```python
from build123d import *

# Parameters (mm, degrees)
SKETCH1_W                    = 443
SKETCH1_H                    = 300
BASE_FLANGE1_DEPTH           = 2
SKETCHED_START               = -221.5
SKETCHED_BEND1_DEPTH         = 443
SKETCHED_BEND1_2_DEPTH       = 443
SKETCHED_BEND2_DEPTH         = 443
SKETCHED_BEND2_2_DEPTH       = 443
EDGE_FLANGE1_STRIP_W         = 10
EDGE_FLANGE1_STRIP_H         = 2
EDGE_FLANGE1_STRIP_CUT_DEPTH = 238.429203673
EDGE_FLANGE1_DEPTH           = 238.429203673
EDGE_FLANGE2_STRIP_W         = 10
EDGE_FLANGE2_STRIP_H         = 2
EDGE_FLANGE2_STRIP_CUT_DEPTH = 238.429203673
EDGE_FLANGE2_DEPTH           = 238.429203673
SKETCH15_W                   = 420
SKETCH15_H                   = 165
CUT_EXTRUDE1_DEPTH           = 272.023210126


# Read off the part's stored shape, not the designer's step: Sketched Bend1, Sketched Bend2
# Sheet-metal steps are written as plain solids
with BuildPart() as part:
    # Sketch1 → Base-Flange1 (new body)
    with BuildSketch(Plane.XY):
        Rectangle(SKETCH1_W, SKETCH1_H)
    extrude(amount=-BASE_FLANGE1_DEPTH)

    # Sketched Bend1 outline → Sketched Bend1 (cut)
    with BuildSketch(Plane.YZ.offset(SKETCHED_START)):
        with BuildLine():
            Line((150, 0), (91.257630798, 0))
            ThreePointArc((91.257630798, 0), (90.161254481, -1.449489743), (88.429203673, -2))
            Line((88.429203673, -2), (150, -2))
            Line((150, -2), (150, 0))
        make_face()
    extrude(amount=SKETCHED_BEND1_DEPTH, mode=Mode.SUBTRACT)

    # Sketched Bend1 2 outline → Sketched Bend1 2 (add)
    with BuildSketch(Plane.YZ.offset(SKETCHED_START)):
        with BuildLine():
            Line((91.429203673, 1), (91.429203673, 59.429203673))
            Line((91.429203673, 59.429203673), (89.429203673, 59.429203673))
            Line((89.429203673, 59.429203673), (89.429203673, 1))
            ThreePointArc((89.429203673, 1), (89.136310454, 0.292893219), (88.429203673, 0))
            Line((88.429203673, 0), (91.257630798, 0))
            ThreePointArc((91.257630798, 0), (91.385999352, 0.492694064), (91.429203673, 1))
        make_face()
    extrude(amount=SKETCHED_BEND1_2_DEPTH)

    # Sketched Bend2 outline → Sketched Bend2 (cut)
    with BuildSketch(Plane.YZ.offset(SKETCHED_START)):
        with BuildLine():
            ThreePointArc((89.429203673, 31.472232635), (90.878693416, 30.375856318), (91.429203673, 28.64380551))
            Line((91.429203673, 28.64380551), (91.429203673, 59.429203673))
            Line((91.429203673, 59.429203673), (89.429203673, 59.429203673))
            Line((89.429203673, 59.429203673), (89.429203673, 31.472232635))
        make_face()
    extrude(amount=SKETCHED_BEND2_DEPTH, mode=Mode.SUBTRACT)

    # Sketched Bend2 2 outline → Sketched Bend2 2 (add)
    with BuildSketch(Plane.YZ.offset(SKETCHED_START)):
        with BuildLine():
            Line((89.429203673, 28.64380551), (89.429203673, 31.472232635))
            ThreePointArc((89.429203673, 31.472232635), (88.936509609, 31.600601189), (88.429203673, 31.64380551))
            Line((88.429203673, 31.64380551), (60.785398163, 31.64380551))
            Line((60.785398163, 31.64380551), (60.785398163, 29.64380551))
            Line((60.785398163, 29.64380551), (88.429203673, 29.64380551))
            ThreePointArc((88.429203673, 29.64380551), (89.136310454, 29.350912291), (89.429203673, 28.64380551))
        make_face()
    extrude(amount=SKETCHED_BEND2_2_DEPTH)

    # Edge-Flange1 strip (across the edge) → Edge-Flange1 strip cut (cut)
    with BuildSketch(Plane(origin=(-221.5, 88.429203673, 0), x_dir=(1, 0, 0), z_dir=(0, -1, 0))):
        with Locations((-4, -1)):
            Rectangle(EDGE_FLANGE1_STRIP_W, EDGE_FLANGE1_STRIP_H)
    extrude(amount=EDGE_FLANGE1_STRIP_CUT_DEPTH, mode=Mode.SUBTRACT)

    # Edge-Flange1 section (across the edge) → Edge-Flange1 (add)
    with BuildSketch(Plane(origin=(-221.5, 88.429203673, 0), x_dir=(1, 0, 0), z_dir=(0, -1, 0))):
        with BuildLine():
            Line((-2, 1), (-2, 10))
            Line((-2, 10), (0, 10))
            Line((0, 10), (0, 1))
            ThreePointArc((0, 1), (0.292893219, 0.292893219), (1, 0))
            Line((1, 0), (1, -2))
            ThreePointArc((1, -2), (-1.121320344, -1.121320344), (-2, 1))
        make_face()
    extrude(amount=EDGE_FLANGE1_DEPTH)

    # Edge-Flange2 strip (across the edge) → Edge-Flange2 strip cut (cut)
    with BuildSketch(Plane(origin=(221.5, -150, 0), x_dir=(-1, 0, 0), z_dir=(0, 1, 0))):
        with Locations((-4, -1)):
            Rectangle(EDGE_FLANGE2_STRIP_W, EDGE_FLANGE2_STRIP_H)
    extrude(amount=EDGE_FLANGE2_STRIP_CUT_DEPTH, mode=Mode.SUBTRACT)

    # Edge-Flange2 section (across the edge) → Edge-Flange2 (add)
    with BuildSketch(Plane(origin=(221.5, -150, 0), x_dir=(-1, 0, 0), z_dir=(0, 1, 0))):
        with BuildLine():
            Line((-2, 1), (-2, 10))
            Line((-2, 10), (0, 10))
            Line((0, 10), (0, 1))
            ThreePointArc((0, 1), (0.292893219, 0.292893219), (1, 0))
            Line((1, 0), (1, -2))
            ThreePointArc((1, -2), (-1.121320344, -1.121320344), (-2, 1))
        make_face()
    extrude(amount=EDGE_FLANGE2_DEPTH)

    # Sketch15 → Cut-Extrude1 (cut, through all)
    with BuildSketch(Plane.XY):
        with Locations((0, -30.864518484)):
            Rectangle(SKETCH15_W, SKETCH15_H)
    extrude(amount=-CUT_EXTRUDE1_DEPTH, mode=Mode.SUBTRACT)


solid = part.part
```
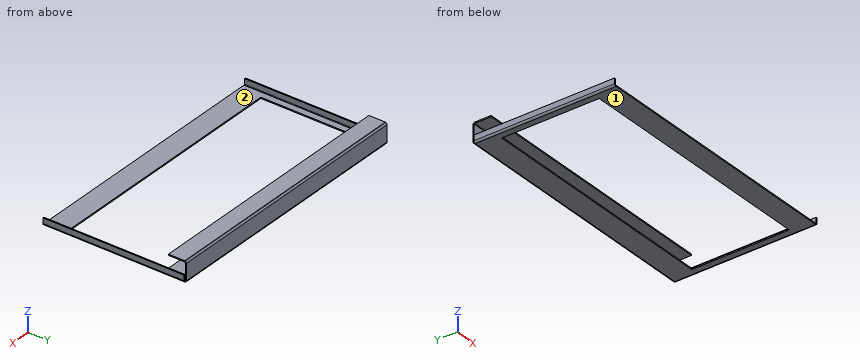
Check sheet for the modelled part. Datum: model origin and axes. Units: mm. Face numbers are marked on the shaded views. Give positions to 0.01 mm unless a question says otherwise; leave off trailing zeros. Order: outer loops, then holes, each group sorted by start corner. A loop starts at its lowest first (then second) coordinate and runs counter-clockwise, first axis right, second up. Notation, with made-up numbers: M 23,65.5 L 32,65.5 A27 cw 32,100.5 Z; hole C -15.5,50 d3. An arc over 180 degrees is marked long. Answer in a Markdown table with one row per item.
1) Cross-section at C-C, the plane y = 74.5. Enter the section's corners in (x, z).
Filled sheet:
| item | result |
|---|---|
| outline | M -223.5,1 A3 ccw -220.5,-2 L 220.5,-2 A3 ccw 223.5,1 L 223.5,10 L 221.5,10 L 221.5,1 A1 cw 220.5,0 L -220.5,0 A1 cw -221.5,1 L -221.5,10 L -223.5,10 Z; M -221.5,29.64 L 221.5,29.64 L 221.5,31.64 L -221.5,31.64 Z |
2) Cross-section at A-A, the plane y = -23.5. Enter the section's corners in (x, z).
Filled sheet:
| item | result |
|---|---|
| outline | M -223.5,1 A3 ccw -220.5,-2 L -210,-2 L -210,0 L -220.5,0 A1 cw -221.5,1 L -221.5,10 L -223.5,10 Z; M 210,-2 L 220.5,-2 A3 ccw 223.5,1 L 223.5,10 L 221.5,10 L 221.5,1 A1 cw 220.5,0 L 210,0 Z |
3) Cross-section at B-B, the plane x = 139. Enter the section's corners in (y, z), plus the area to 3 significant figures.
Filled sheet:
| item | result |
|---|---|
| outline | M -150,-2 L -113.36,-2 L -113.36,0 L -150,0 Z; M 51.64,-2 L 88.43,-2 A3 ccw 91.43,1 L 91.43,28.64 A3 ccw 88.43,31.64 L 60.79,31.64 L 60.79,29.64 L 88.43,29.64 A1 cw 89.43,28.64 L 89.43,1 A1 cw 88.43,0 L 51.64,0 Z |
| area | 270 mm2 |
4) Thickness scan on L1, parallel to X at y = -121.5, z = 5.5; L2, parallel to Y at x = -187, z = 12; L3, parallel to Z at x = 116, y = -132. Record the ranges inside material, lowest first. Write a range as [from, to].
Filled sheet:
| item | result |
|---|---|
| L1 | x = [-223.5, -221.5], [221.5, 223.5] |
| L2 | y = [89.43, 91.43] |
| L3 | z = [-2, 0] |
5) Release check for a two-part mould opening along X. For the marked faces 1 and 2 record: +X half, -X half, draft (parallel to the pull), parting line (faces both ways), or undercut.
Filled sheet:
| item | result |
|---|---|
| face 1 | draft |
| face 2 | undercut |
6) Cross-section at D-D, the plane z = 24.5. Enter the section's corners in (x, y), plus the area to 3 significant figures.
Filled sheet:
| item | result |
|---|---|
| outline | M -221.5,89.43 L 221.5,89.43 L 221.5,91.43 L -221.5,91.43 Z |
| area | 886 mm2 |
7) Gauge pin test, flat ends, axial feed: P1, Ø2, axis at x = -106, z = 3, coming from the -Y side; P2, Ø1, axis at x = -223, y = -79.5, coming from the +Z side; P3, Ø10, axis at y = 21, z = 18.5, coming from the +X side; P4, Ø2, axis at x = 54, z = -1, coming from the +Y side. Record the tip position at first contact, or that the pin passes through.
Filled sheet:
| item | result |
|---|---|
| P1 | stops at y = 89.43 |
| P2 | stops at z = 10 |
| P3 | passes through |
| P4 | stops at y = 91.26 |
